```python
from build123d import *

# Parameters (mm, degrees)
SKETCH3_W           = 30
SKETCH3_H           = 45
BOSS_EXTRUDE1_DEPTH = 15
SKETCH4_W           = 20
SKETCH4_H           = 15
BOSS_EXTRUDE2_DEPTH = 15
SKETCH5_W           = 20
SKETCH5_H           = 15
BOSS_EXTRUDE3_DEPTH = 8
FILLET1_R           = 2
SKETCH6_R           = 5
BOSS_EXTRUDE4_DEPTH = 2
SKETCH7_R           = 2.5
BOSS_EXTRUDE5_DEPTH = 6.5


with BuildPart() as part:
    # Sketch3 → Boss-Extrude1 (new body)
    with BuildSketch(Plane.XY):
        with Locations((-15, 22.5)):
            Rectangle(SKETCH3_W, SKETCH3_H)
    extrude(amount=BOSS_EXTRUDE1_DEPTH)

    # Sketch4 → Boss-Extrude2 (add)
    with BuildSketch(Plane.XY.offset(15)):
        with Locations((-15, 32.5)):
            Rectangle(SKETCH4_W, SKETCH4_H)
    extrude(amount=BOSS_EXTRUDE2_DEPTH)

    # Sketch5 → Boss-Extrude3 (add)
    with BuildSketch(Plane(origin=(0, 0, 0), x_dir=(-1, 0, 0), z_dir=(0, 0, -1))):
        with Locations((15, 32.5)):
            Rectangle(SKETCH5_W, SKETCH5_H)
    extrude(amount=BOSS_EXTRUDE3_DEPTH)

    # Fillet1
    fillet1_edges = [part.edges().sort_by_distance(p)[0] for p in [
        (-25, 40, 22.5),
        (-25, 25, 22.5),
        (-5, 25, 22.5),
        (-5, 40, 22.5),
        (-5, 40, -4),
        (-5, 25, -4),
        (-25, 25, -4),
        (-25, 40, -4),
    ]]
    fillet(fillet1_edges, radius=FILLET1_R)

    # Sketch6 → Boss-Extrude4 (add)
    with BuildSketch(Plane.XY.offset(30)):
        with Locations((-15, 32.5)):
            Circle(SKETCH6_R)
    extrude(amount=BOSS_EXTRUDE4_DEPTH)

    # Sketch7 → Boss-Extrude5 (add)
    with BuildSketch(Plane.XY.offset(32)):
        with Locations(Location((-15, 32.5, 0), (0, 0, 180))):
            Circle(SKETCH7_R)
    extrude(amount=BOSS_EXTRUDE5_DEPTH)


solid = part.part
```
CAD build for the part. Positions are in the model's coordinates, mm. A direction names the side the tool comes from. Coordinates: 2 decimals unless noted, no trailing zeros. Loops run counter-clockwise (first coordinate to the right, second up) from the corner with the lowest first, then second, coordinate; pieces in that order, holes last. Notation, with made-up numbers: (12.5, 77) - (24.5, 77) arc R13 cw to (24.5, 98) - close; hole circle Ø5 at (39, 54). An arc over 180 degrees is marked (long way). Use CSV: the item, a comma, the result in double quotes. Start each with the question number.
Q1. Drop flat-ended pins along their axis: P1, Ø9, axis at y = 32, z = 23.5, coming from the -X side; P2, Ø2.5, axis at x = -12.5, z = -4.5, coming from the -Y side; P3, Ø6.5, axis at x = -12, z = -5.5, coming from the +Y side. Give the stop position or say it passes through.
Q2. Cut at A-A, the plane x = -15. List the corners of the cut face in (y, z), then the cut area to 3 significant figures.
Q3. Probe probe 1 along Z at (x, y) = (-5.5, 36.5); probe 2 along Z at (x, y) = (-25, 2); probe 3 along Y at (x, z) = (-9, 22.5). List the from-to ranges inside material, lowest first. Write a range as from..to.
Q4. Two-plate mould, pull along X, no slides. Class faces 1 (the flat face through (-15, 18, 0)), 2 (the cylindrical face through (-5.57, 39.4, 22.6)), 3 (the cylindrical face through (-24.4, 25.57, 22.6)): +X half, -X half, draft (parallel to the pull), parting line (faces both ways), or undercut.
Q5. Cut at D-D, the plane x = -18.5. List the corners of the cut face in (y, z), then the cut area to 3 significant figures.
Q6. 3-axis set-ups, long thin cutter, end or side, ignore diameter. For faces 4 (the flat face through (-25, 32, -4)), 5 (the flat face through (-5, 32, 22)), 6 (the flat face through (-15, 25, 22)), 7 (the cylindrical face through (-24.4, 39.43, 22.6)), 8 (the cylindrical face through (-19.995, 32.72, 30.986)): which of +Z, -Z, +X, -X, +Y, -Y reach the whole face in a straight line?
Q7. Cut at B-B, the plane z = -3. List the corners of the cut face in (x, y), then the cut area to 3 significant figures.
Q8. Cut at C-C, the plane y = 32.5. List the corners of the cut face in (x, z).
Here are the results:
1,P1,"x = -25"
1,P2,"y = 25"
1,P3,"y = 40"
2,outline,"(0, 0) - (25, 0) - (25, -8) - (40, -8) - (40, 0) - (45, 0) - (45, 15) - (40, 15) - (40, 30) - (37.5, 30) - (37.5, 32) - (35, 32) - (35, 38.5) - (30, 38.5) - (30, 32) - (27.5, 32) - (27.5, 30) - (25, 30) - (25, 15) - (0, 15) - close"
2,area,"1,070 mm2"
3,probe 1,"-8..30"
3,probe 2,"0..15"
3,probe 3,"25..40"
4,face 1,"draft"
4,face 2,"+X half"
4,face 3,"-X half"
5,outline,"(0, 0) - (25, 0) - (25, -8) - (40, -8) - (40, 0) - (45, 0) - (45, 15) - (40, 15) - (40, 30) - (36.07, 30) - (36.07, 32) - (28.93, 32) - (28.93, 30) - (25, 30) - (25, 15) - (0, 15) - close"
5,area,"1,030 mm2"
6,face 4,"-Z, -X, +Y, -Y"
6,face 5,"+Z, +X, +Y, -Y"
6,face 6,"+Z, +X, -X, -Y"
6,face 7,"+Z, -X, +Y"
6,face 8,"+Z"
7,outline,"(-25, 27) arc R2 ccw to (-23, 25) - (-7, 25) arc R2 ccw to (-5, 27) - (-5, 38) arc R2 ccw to (-7, 40) - (-23, 40) arc R2 ccw to (-25, 38) - close"
7,area,"297 mm2"
8,outline,"(-30, 0) - (-25, 0) - (-25, -8) - (-5, -8) - (-5, 0) - (0, 0) - (0, 15) - (-5, 15) - (-5, 30) - (-10, 30) - (-10, 32) - (-12.5, 32) - (-12.5, 38.5) - (-17.5, 38.5) - (-17.5, 32) - (-20, 32) - (-20, 30) - (-25, 30) - (-25, 15) - (-30, 15) - close"
